from build123d import *

# Parameters (mm, degrees)
BOSS_EXTRUDE1_DEPTH                                 = 4.5
CUT_EXTRUDE1_DEPTH                                  = 43.552908244
CUT_EXTRUDE1_DEPTH_BACK                             = 43.552908244
SKETCH2_W                                           = 4.5
SKETCH2_H                                           = 2.3
CUT_EXTRUDE2_DEPTH                                  = 34.234018716
CUT_EXTRUDE2_DEPTH_BACK                             = 34.234018716
CBORE_FOR_M3_HEX_SOCKET_HEAD_CAP_SCREW1_D           = 3.6
CBORE_FOR_M3_HEX_SOCKET_HEAD_CAP_SCREW1_CBORE_D     = 6.5
CBORE_FOR_M3_HEX_SOCKET_HEAD_CAP_SCREW1_CBORE_DEPTH = 3.4
FILLET2_DEPTH                                       = 4.5
FILLET2_2_DEPTH                                     = 2.2
CHAMFER1_SIZE                                       = 3
CHAMFER2_SIZE                                       = 2


with BuildPart() as part:
    # Sketch1 → Boss-Extrude1 (new body)
    with BuildSketch(Plane(origin=(0, 0, 0), x_dir=(1, 0, 0), z_dir=(0, 1, 0))):
        with BuildLine():
            Line((-18.10386699, 12.5), (-24.5, 12.5))
            Line((-24.5, 12.5), (-24.5, -12.5))
            Line((-24.5, -12.5), (-18.10386699, -12.5))
            ThreePointArc((-18.10386699, -12.5), (22, 0), (-18.10386699, 12.5))
        make_face()
    extrude(amount=BOSS_EXTRUDE1_DEPTH)

    # Sketch2 → Cut-Extrude1 (cut, two sides: drawn at the far end of the back side and taken through both)
    with BuildSketch(Plane.XY.offset(12.5).offset(-CUT_EXTRUDE1_DEPTH_BACK)):
        with Locations((-22.25, 3.35)):
            Rectangle(SKETCH2_W, SKETCH2_H)
    extrude(amount=CUT_EXTRUDE1_DEPTH + CUT_EXTRUDE1_DEPTH_BACK, mode=Mode.SUBTRACT)

    # Sketch3 → Cut-Extrude2 (cut, two sides: drawn at the far end of the back side and taken through both)
    with BuildSketch(Plane(origin=(0, 4.5, 0), x_dir=(1, 0, 0), z_dir=(0, 1, 0)).offset(-CUT_EXTRUDE2_DEPTH_BACK)):
        with BuildLine():
            Line((0, 6), (-24.5, 6))
            Line((-24.5, 6), (-24.5, -6))
            Line((-24.5, -6), (0, -6))
            ThreePointArc((0, -6), (6, 0), (0, 6))
        make_face()
    extrude(amount=CUT_EXTRUDE2_DEPTH + CUT_EXTRUDE2_DEPTH_BACK, mode=Mode.SUBTRACT)

    # CBORE for M3 Hex Socket Head Cap Screw1 (through all)
    with Locations(Plane(origin=(0, 4.5, 0), x_dir=(1, 0, 0), z_dir=(0, 1, 0))):
        with Locations((0, -17.5), (0, 17.5)):
            CounterBoreHole(CBORE_FOR_M3_HEX_SOCKET_HEAD_CAP_SCREW1_D / 2, CBORE_FOR_M3_HEX_SOCKET_HEAD_CAP_SCREW1_CBORE_D / 2, CBORE_FOR_M3_HEX_SOCKET_HEAD_CAP_SCREW1_CBORE_DEPTH)

    # Fillet2: read off the stored shape, not the designer's step
    # Fillet2 outline → Fillet2 (add)
    with BuildSketch(Plane(origin=(0, 0, 0), x_dir=(1, 0, 0), z_dir=(0, 1, 0))):
        with BuildLine():
            Line((-18.10386699, -12.5), (-20, -12.5))
            Line((-20, -12.5), (-20, -13.548778219))
            ThreePointArc((-20, -13.548778219), (-16.860589429, -14.993334166), (-14.016717362, -16.956757779))
            ThreePointArc((-14.016717362, -16.956757779), (-16.214149909, -14.869476882), (-18.10386699, -12.5))
        make_face()
        with BuildLine():
            ThreePointArc((-18.10386699, 12.5), (-16.214149909, 14.869476882), (-14.016717362, 16.956757779))
            ThreePointArc((-14.016717362, 16.956757779), (-16.860589429, 14.993334166), (-20, 13.548778219))
            Line((-20, 13.548778219), (-20, 12.5))
            Line((-20, 12.5), (-18.10386699, 12.5))
        make_face()
    extrude(amount=FILLET2_DEPTH)

    # Fillet2 2 outline → Fillet2 2 (add)
    with BuildSketch(Plane(origin=(0, 0, 0), x_dir=(1, 0, 0), z_dir=(0, 1, 0))):
        with BuildLine():
            Line((-20, -13.548778219), (-20, -12.5))
            Line((-20, -12.5), (-24.5, -12.5))
            ThreePointArc((-24.5, -12.5), (-22.219610886, -12.893998326), (-20, -13.548778219))
        make_face()
        with BuildLine():
            Line((-20, 12.5), (-20, 13.548778219))
            ThreePointArc((-20, 13.548778219), (-22.219610886, 12.893998326), (-24.5, 12.5))
            Line((-24.5, 12.5), (-20, 12.5))
        make_face()
    extrude(amount=FILLET2_2_DEPTH)

    # Chamfer1
    chamfer1_edges = [part.edges().sort_by_distance(p)[0] for p in [
        (-10, 4.5, 6),
        (-10, 4.5, -6),
        (6, 4.5, 0),
    ]]
    chamfer(chamfer1_edges, length=CHAMFER1_SIZE)

    # Chamfer2
    # the kernel refuses this chamfer: 2 mm, written as the material it takes off along each edge
    with BuildSketch(Plane(origin=(0, 4.5, 0), x_dir=(-0.6371235164664789, 0, 0.7707617172417092), z_dir=(-0.7707617172417092, 0, -0.6371235164664789))) as chamfer2_piece_1:
        Polygon((22 - CHAMFER2_SIZE, 0), (22, -CHAMFER2_SIZE), (22, 0), align=None)
    revolve(axis=Axis((0, 4.5, 0), (0, 1, 0)), revolution_arc=259.155320495, mode=Mode.SUBTRACT)
    with BuildSketch(Plane(origin=(-26.75918769, 4.5, -32.371992129), x_dir=(0.6371235163113105, 0, 0.7707617173699738), z_dir=(0.7707617173699738, 0, -0.6371235163113105))) as chamfer2_piece_2:
        Polygon((20.000000004, CHAMFER2_SIZE), (20.000000004 + CHAMFER2_SIZE, 0), (20.000000004, 0), align=None)
    revolve(axis=Axis((-26.75918769, 4.5, -32.371992129), (0, -1, 0)), revolution_arc=34.56000809, mode=Mode.SUBTRACT)
    with BuildSketch(Plane(origin=(-26.75918769, 4.5, 32.371992129), x_dir=(0.08746265429711, 0, -0.9961677991700516), z_dir=(-0.9961677991700516, 0, -0.08746265429711))) as chamfer2_piece_3:
        Polygon((20.000000004 + CHAMFER2_SIZE, 0), (20.000000004, CHAMFER2_SIZE), (20.000000004, 0), align=None)
    revolve(axis=Axis((-26.75918769, 4.5, 32.371992129), (0, -1, 0)), revolution_arc=34.56000809, mode=Mode.SUBTRACT)


solid = part.part
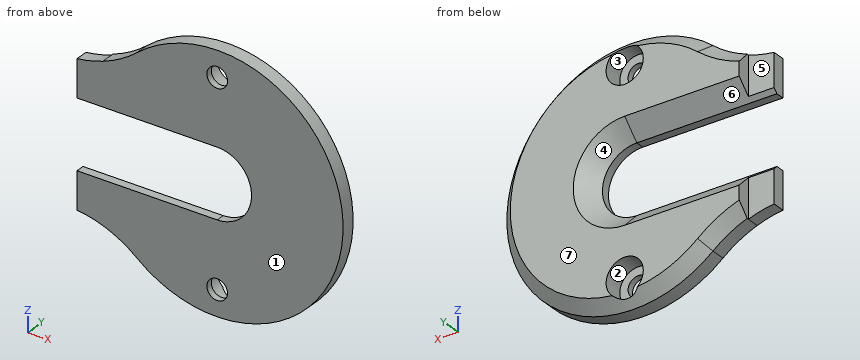
CAD build for the part. Positions are in the model's coordinates, mm. Face numbers are marked on the shaded views. A direction names the side the tool comes from. Give positions to 0.01 mm unless a question says otherwise; leave off trailing zeros. Write each loop counter-clockwise with the first axis right and the second up, starting at its lowest first coordinate (ties: lowest second). Pieces come first, ordered by that corner, then holes. Notation, with made-up numbers: (-22.75, 16.25) -> (22.25, 16.25) arc R18 cw to (22.25, 20.25) -> close; hole circle Ø5 at (55.25, 82). An arc over 180 degrees is marked (long way). Return JSON: item names as keys, results as strings.
Item 1: Band-saw the part on A-A (y = 3.4). List the corners of the cut face in (x, z).
Answer below:
{"outline": "(-20, -12.6) arc R20.9 cw to (-13.44, -16.26) arc R21.1 ccw (long way) to (-13.44, 16.26) arc R20.9 cw to (-20, 12.6) -> (-20, 7.9) -> (0, 7.9) arc R7.9 cw to (0, -7.9) -> (-20, -7.9) -> close; hole circle Ø6.5 at (0, -17.5); hole circle Ø6.5 at (0, 17.5)"}
Item 2: Band-saw the part on C-C (x = -1). Give the number of separate pieces and of enclosed holes in the cut face, then the cut area to 3 significant figures.
Answer below:
{"separate pieces": "4", "enclosed holes": "0", "area": "82.5 mm2"}
Item 3: Drop flat-ended pins along their axis: pin 1 (1.5 mm diameter, centred on x = 9.5, y = 1.5, fed in from -Z); pin 2 (0.8 mm diameter, centred on x = -15.5, y = 0.5, fed in from +Z); pin 3 (5 mm diameter, centred on x = -0.5, z = -18, fed in from +Y). Give the stop position or say it passes through.
Answer below:
{"pin 1": "stops at z = -20.19", "pin 2": "stops at z = 16.12", "pin 3": "stops at y = 1.1"}
Item 4: Tool access for the marked faces 5, 6 and 7: list every direction of +Z, -Z, +X, -X, +Y, -Y with a clear straight run to the whole face (end or side of a thin tool).
Answer below:
{"face 5": "+Z, -Z, -X, +Y", "face 6": "-X, +Y", "face 7": "+Z, -Z, +X, -X, +Y"}
Item 5: Drill centre lines: probe 1 along Z at (x, y) = (0, 0.6); probe 2 along Z at (x, y) = (2.5, 4.3); probe 3 along X at (y, z) = (4.3, -17.5). Where is each one in solid material? Low to high.
Answer below:
{"probe 1": "z = -22 to -19.3, -15.7 to -6, 6 to 15.7, 19.3 to 22", "probe 2": "z = -20.04 to -19.58, -15.42 to -8.44, 8.44 to 15.42, 19.58 to 20.04", "probe 3": "x = -10.09 to -3.25, 3.25 to 10.09"}
Item 6: Band-saw the part on B-B (z = 0). List the corners of the cut face in (x, y).
Answer below:
{"outline": "(6, 0) -> (22, 0) -> (22, 2.5) -> (20, 4.5) -> (9, 4.5) -> (6, 1.5) -> close"}
Item 7: Two-plate mould, pull along X, no slides. Class the marked faces 1, 2, 3 and 4: +X half, -X half, draft (parallel to the pull), parting line (faces both ways), or undercut.
Answer below:
{"face 1": "draft", "face 2": "undercut", "face 3": "undercut", "face 4": "-X half"}
